```python
from build123d import *

# Parameters (mm, degrees)
PAD_DEPTH            = 7
SKETCH001_W          = 1
SKETCH001_H          = 24.5
POCKET_DEPTH         = 7.001
POCKET_DEPTH_BACK    = -7.001
SKETCH002_R          = 6
POCKET001_DEPTH      = 7.001
POCKET001_DEPTH_BACK = -7.001
SKETCH003_R          = 2.75
POCKET002_DEPTH      = 0.001
POCKET002_DEPTH_BACK = -37.501
SKETCH004_R          = 2.25
POCKET003_DEPTH      = 21.001
POCKET003_DEPTH_BACK = -21.001
SKETCH005_R          = 3.75
POCKET004_DEPTH      = 4.5


with BuildPart() as part:
    # Sketch → Pad (new body, symmetric)
    with BuildSketch(Plane.XZ):
        Polygon((-21, 0), (21, 0), (21, 6), (10, 6), (10, 37.5), (-10, 37.5), (-10, 6), (-21, 6), align=None)
    extrude(amount=PAD_DEPTH, both=True)

    # Sketch001 → Pocket (cut, two sides)
    with BuildSketch(Plane.XZ) as pocket_sk:
        with Locations((0, 35.25)):
            Rectangle(SKETCH001_W, SKETCH001_H)
    extrude(amount=-POCKET_DEPTH, mode=Mode.SUBTRACT)
    extrude(pocket_sk.sketch, amount=-POCKET_DEPTH_BACK, mode=Mode.SUBTRACT)

    # Sketch002 → Pocket001 (cut, two sides)
    with BuildSketch(Plane.XZ) as pocket001_sk:
        with Locations((0, 23)):
            Circle(SKETCH002_R)
    extrude(amount=-POCKET001_DEPTH, mode=Mode.SUBTRACT)
    extrude(pocket001_sk.sketch, amount=-POCKET001_DEPTH_BACK, mode=Mode.SUBTRACT)

    # Sketch003 → Pocket002 (cut, two sides)
    with BuildSketch(Plane.XY) as pocket002_sk:
        with Locations((-16, 0)):
            Circle(SKETCH003_R)
        with Locations((16, 0)):
            Circle(SKETCH003_R)
    extrude(amount=-POCKET002_DEPTH, mode=Mode.SUBTRACT)
    extrude(pocket002_sk.sketch, amount=-POCKET002_DEPTH_BACK, mode=Mode.SUBTRACT)

    # Sketch004 → Pocket003 (cut, two sides)
    with BuildSketch(Plane.YZ) as pocket003_sk:
        with Locations((0, 33)):
            Circle(SKETCH004_R)
    extrude(amount=-POCKET003_DEPTH, mode=Mode.SUBTRACT)
    extrude(pocket003_sk.sketch, amount=-POCKET003_DEPTH_BACK, mode=Mode.SUBTRACT)

    # Sketch005 (on Face16 of Pocket003) → Pocket004 (cut)
    with BuildSketch(Plane(origin=(10, 0, 0), x_dir=(0, 0, 1), z_dir=(1, 0, 0))):
        with Locations((33, 0)):
            Circle(SKETCH005_R)
    extrude(amount=-POCKET004_DEPTH, mode=Mode.SUBTRACT)


solid = part.part
```
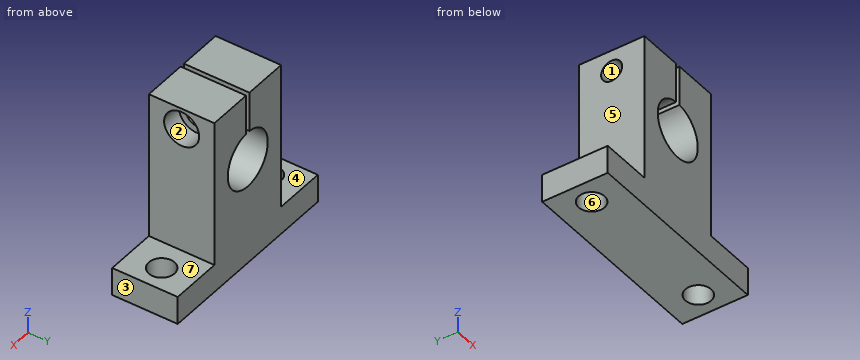
Part model, mm, in its own coordinate system. Face numbers are marked on the shaded views. A direction names the side the tool comes from. Round coordinates to 2 decimals unless told otherwise and drop trailing zeros. Order: outer loops, then holes, each group sorted by start corner. A loop starts at its lowest first (then second) coordinate and runs counter-clockwise, first axis right, second up. Notation, with made-up numbers: M -12,12 L 36,12 A19 ccw 36,42 Z; hole C 60,22.25 d5. An arc over 180 degrees is marked long. Answer in a Markdown table with one row per item. Add a question column.
Q1. Wall check: L1, parallel to X at y = 0, z = 4; L2, parallel to X at y = -1, z = 23; L3, parallel to Y at x = 8, z = 33. Give the ranges that are in metal, low to high. Write a range as from..to.
Q2. Cut at B-B on z = 33. Give the cut face in (x, y).
Q3. Cut at C-C on y = 0. Give the number of separate pieces and of enclosed holes in the cut face, and give its area (3 significant figures).
Q4. Mould opens along Z. For the marked faces 1, 2, 3 and 4 say: +Z half, -Z half, draft (parallel to the pull), parting line (faces both ways), or undercut.
Q5. Cut at A-A on x = -16. Give the cut face in (y, z).
Q6. Cut at D-D on z = 23. Give the cut face in (x, y).
Q7. Pin check, flat tips, straight feed: pin 1 (3 mm diameter, centred on y = -1, z = 20.5, fed in from +X); pin 2 (2.5 mm diameter, centred on y = 0, z = 33, fed in from -X); pin 3 (6 mm diameter, centred on y = 0, z = 33, fed in from -X); pin 4 (5.5 mm diameter, centred on x = -17, y = 0, fed in from +Z). Stop position of each tip, or through.
Q8. 3-axis set-ups, long thin cutter, end or side, ignore diameter. For the marked faces 5, 6 and 7: which of +Z, -Z, +X, -X, +Y, -Y reach the whole face in a straight line?
Established:
| question | item | result |
|---|---|---|
| 1 | L1 | x = -21..-18.75, -13.25..13.25, 18.75..21 |
| 1 | L2 | x = -10..-6, 6..10 |
| 1 | L3 | y = -7..-3.75, 3.75..7 |
| 2 | outline | M -10,-7 L -0.5,-7 L -0.5,-2.25 L -10,-2.25 Z; M -10,2.25 L -0.5,2.25 L -0.5,7 L -10,7 Z; M 0.5,-7 L 10,-7 L 10,-3.75 L 5.5,-3.75 L 5.5,-2.25 L 0.5,-2.25 Z; M 0.5,2.25 L 5.5,2.25 L 5.5,3.75 L 10,3.75 L 10,7 L 0.5,7 Z |
| 3 | separate pieces | 5 |
| 3 | enclosed holes | 0 |
| 3 | area | 595 mm2 |
| 4 | face 1 | undercut |
| 4 | face 2 | undercut |
| 4 | face 3 | draft |
| 4 | face 4 | +Z half |
| 5 | outline | M -7,0 L -2.75,0 L -2.75,6 L -7,6 Z; M 2.75,0 L 7,0 L 7,6 L 2.75,6 Z |
| 6 | outline | M -10,-7 L -6,-7 L -6,7 L -10,7 Z; M 6,-7 L 10,-7 L 10,7 L 6,7 Z |
| 7 | pin 1 | stops at x = 10 |
| 7 | pin 2 | passes through |
| 7 | pin 3 | stops at x = -10 |
| 7 | pin 4 | stops at z = 6 |
| 8 | face 5 | +Z, -X, +Y, -Y |
| 8 | face 6 | +Z, -Z |
| 8 | face 7 | +Z, +X, +Y, -Y |
